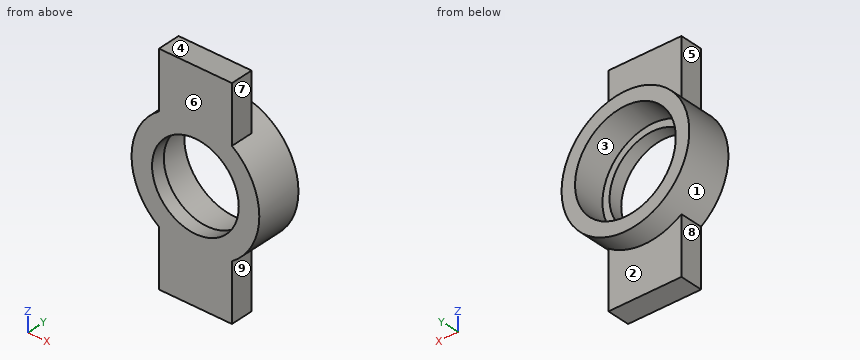
from build123d import *

# Parameters (mm, degrees)
SKETCH1_R           = 14
SKETCH1_R_2         = 11.05
BOSS_EXTRUDE1_DEPTH = 10
SKETCH1_3_R         = 11.05
SKETCH1_3_R_2       = 9.5
BOSS_EXTRUDE2_DEPTH = 3
BOSS_EXTRUDE3_START = -2.510875
SKETCH4_W           = 16
SKETCH4_H           = 5.016393312
BOSS_EXTRUDE3_DEPTH = 12.510875


with BuildPart() as part:
    # Sketch1 → Boss-Extrude1 (new body)
    with BuildSketch(Plane(origin=(0, 0, 0), x_dir=(1, 0, 0), z_dir=(0, 1, 0))):
        Circle(SKETCH1_R)
        Circle(SKETCH1_R_2, mode=Mode.SUBTRACT)
    extrude(amount=BOSS_EXTRUDE1_DEPTH)

    # Sketch1<3> → Boss-Extrude2 (add)
    with BuildSketch(Plane(origin=(0, 0, 0), x_dir=(1, 0, 0), z_dir=(0, 1, 0))):
        Circle(SKETCH1_3_R)
        Circle(SKETCH1_3_R_2, mode=Mode.SUBTRACT)
    extrude(amount=BOSS_EXTRUDE2_DEPTH)

    # Sketch4 → Boss-Extrude3 (add)
    with BuildSketch(Plane.XY.offset(14).offset(BOSS_EXTRUDE3_START)):
        with Locations((0, 2.508196656)):
            Rectangle(SKETCH4_W, SKETCH4_H)
    boss_extrude3 = extrude(amount=BOSS_EXTRUDE3_DEPTH)

    # Mirror1: Boss-Extrude3 across plane
    add(boss_extrude3.mirror(Plane.XY))


solid = part.part
The listing builds one solid part. Answer for the finished solid, in the listing's coordinates (mm). Face numbers are marked on the shaded views. A direction names the side the tool comes from. Give positions to 0.01 mm unless a question says otherwise; leave off trailing zeros. Order: outer loops, then holes, each group sorted by start corner. A loop starts at its lowest first (then second) coordinate and runs counter-clockwise, first axis right, second up. Notation, with made-up numbers: (2, 79) - (32, 79) arc R12 ccw to (32, 88) - close; hole circle Ø8 at (9, -21). An arc over 180 degrees is marked (long way). Answer as CSV lines item,"result".
Q1. A cutting plane is placed at A-A, the plane z = 0. Determine the outline of the cut face in (x, y), and give its area (3 significant figures).
Answer key:
outline,"(-14, 0) - (-9.5, 0) - (-9.5, 3) - (-11.05, 3) - (-11.05, 10) - (-14, 10) - close; (9.5, 0) - (14, 0) - (14, 10) - (11.05, 10) - (11.05, 3) - (9.5, 3) - close"
area,"68.3 mm^2"
Q2. Each of these flat-tipped pins is pushed along its axis until it touches: pin 1 Ø3 at (x, z) = (6.5, -15.5) entering from +Y; pin 2 Ø10 at (x, z) = (-11, -7) entering from -Y; pin 3 Ø1.5 at (y, z) = (2, 19) entering from +X; pin 4 Ø4 at (x, y) = (-2, 8) entering from -Z. Where does it stop, or does it pass through?
Answer key:
pin 1,"stops at y = 5.02"
pin 2,"stops at y = 0"
pin 3,"stops at x = 8"
pin 4,"stops at z = -14"
Q3. A cutting plane is placed at B-B, the plane y = 1.75. Determine the outline of the cut face in (x, z), and give its area (3 significant figures).
Answer key:
outline,"(-8, -24) - (8, -24) - (8, -11.49) arc R14 ccw to (8, 11.49) - (8, 24) - (-8, 24) - (-8, 11.49) arc R14 ccw to (-8, -11.49) - close; hole circle Ø19 at (0, 0)"
area,"678 mm^2"
Q4. Straight lines are drawn through the part: L1, parallel to X at y = 7.75, z = 0; L2, parallel to Z at x = 0, y = 1.95; L3, parallel to X at y = 0.9, z = 0. For each, find the intervals that lie inside material, in ascending order.
Answer key:
L1,"x = -14 to -11.05, 11.05 to 14"
L2,"z = -24 to -9.5, 9.5 to 24"
L3,"x = -14 to -9.5, 9.5 to 14"
Q5. A cutting plane is placed at D-D, the plane z = -8. Determine the outline of the cut face in (x, y), and give its area (3 significant figures).
Answer key:
outline,"(-11.49, 0) - (-5.12, 0) - (-5.12, 3) - (-7.62, 3) - (-7.62, 10) - (-11.49, 10) - close; (5.12, 0) - (11.49, 0) - (11.49, 10) - (7.62, 10) - (7.62, 3) - (5.12, 3) - close"
area,"92.3 mm^2"
Q6. A cutting plane is placed at C-C, the plane x = 0. Determine the outline of the cut face in (y, z), and give its area (3 significant figures).
Answer key:
outline,"(0, -24) - (5.02, -24) - (5.02, -14) - (10, -14) - (10, -11.05) - (3, -11.05) - (3, -9.5) - (0, -9.5) - close; (0, 9.5) - (3, 9.5) - (3, 11.05) - (10, 11.05) - (10, 14) - (5.02, 14) - (5.02, 24) - (0, 24) - close"
area,"169 mm^2"
Q7. Determine the mould class of the marked faces 1, 2, 3 and 4 for opening direction Z: pulls with the +Z half, pulls with the -Z half, needs draft (parallel to the pull), parting line crosses it, or undercut.
Answer key:
face 1,"parting line crosses it"
face 2,"needs draft"
face 3,"undercut"
face 4,"pulls with the +Z half"
Q8. Which of the six approach directions +Z, -Z, +X, -X, +Y, -Y give full straight-line access (tool end or side, diameter ignored) to the marked faces 5, 6, 7, 8 and 9?
Answer key:
face 5,"+Z, -X, +Y, -Y"
face 6,"+Z, -Z, +X, -X, -Y"
face 7,"+Z, +X, +Y, -Y"
face 8,"-Z, -X, +Y, -Y"
face 9,"-Z, +X, +Y, -Y"
